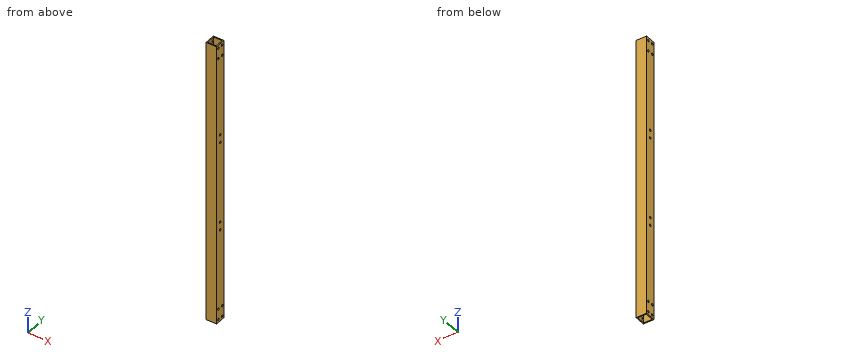
from build123d import *

# Parameters (mm, degrees)
SKETCH_1_W          = 20
SKETCH_1_H          = 20
SKETCH_1_W_2        = 16
SKETCH_1_H_2        = 16
EXTRUDE_1_DEPTH     = 560
SKETCH_2_W          = 20
SKETCH_2_H          = 20
CUT_EXTRUDE_1_DEPTH = 10
SKETCH_3_R          = 2.1
SKETCH_3_R_2        = 2.035272785
CUT_EXTRUDE_2_DEPTH = 551.454357781
SKETCH_4_R          = 2.1
CUT_EXTRUDE_3_DEPTH = 551.454357781


with BuildPart() as part:
    # 草图1 → 凸台-拉伸1 (new body)
    with BuildSketch(Plane.XY):
        Rectangle(SKETCH_1_W, SKETCH_1_H)
        Rectangle(SKETCH_1_W_2, SKETCH_1_H_2, mode=Mode.SUBTRACT)
    extrude(amount=EXTRUDE_1_DEPTH)

    # 草图2 → 切除-拉伸1 (cut)
    with BuildSketch(Plane(origin=(0, 0, 0), x_dir=(-1, 0, 0), z_dir=(0, 0, -1))):
        Rectangle(SKETCH_2_W, SKETCH_2_H)
    cut_extrude_1 = extrude(amount=-CUT_EXTRUDE_1_DEPTH, mode=Mode.SUBTRACT)

    # 镜向1: 切除-拉伸1 across plane
    add(cut_extrude_1.mirror(Plane(origin=(-40, 280, 280), x_dir=(1, 0, 0), z_dir=(0, 0, 1))), mode=Mode.SUBTRACT)

    # 草图3 → 切除-拉伸2 (cut, through all)
    with BuildSketch(Plane(origin=(10, 0, 0), x_dir=(0, 0, -1), z_dir=(1, 0, 0))):
        with Locations((-16, 5)):
            Circle(SKETCH_3_R)
        with Locations((-16, -5)):
            Circle(SKETCH_3_R_2)
        with Locations((-36, 5)):
            Circle(SKETCH_3_R)
        with Locations((-36, -5)):
            Circle(SKETCH_3_R)
        with Locations((-544, 5)):
            Circle(SKETCH_3_R)
        with Locations((-544, -5)):
            Circle(SKETCH_3_R_2)
        with Locations((-524, -5)):
            Circle(SKETCH_3_R)
        with Locations((-524, 5)):
            Circle(SKETCH_3_R)
    extrude(amount=-CUT_EXTRUDE_2_DEPTH, mode=Mode.SUBTRACT)

    # 草图4 → 切除-拉伸3 (cut, through all)
    with BuildSketch(Plane(origin=(10, 0, 0), x_dir=(0, 0, -1), z_dir=(1, 0, 0))):
        with Locations((-187.5, 0)):
            Circle(SKETCH_4_R)
        with Locations((-202.5, 0)):
            Circle(SKETCH_4_R)
        with Locations((-357.5, 0)):
            Circle(SKETCH_4_R)
        with Locations((-372.5, 0)):
            Circle(SKETCH_4_R)
    extrude(amount=-CUT_EXTRUDE_3_DEPTH, mode=Mode.SUBTRACT)


solid = part.part
Check sheet for the modelled part. Datum: model origin and axes. Units: mm. Give positions to 0.01 mm unless a question says otherwise; leave off trailing zeros. Write each loop counter-clockwise with the first axis right and the second up, starting at its lowest first coordinate (ties: lowest second). Pieces come first, ordered by that corner, then holes. Notation, with made-up numbers: (4, 56) -> (30, 56) arc R14 ccw to (30, 83) -> close; hole circle Ø7 at (44, 19.5). An arc over 180 degrees is marked (long way). Write item = value, one per line.
Item 1: Scan lines: probe 1 along Y at (x, z) = (-9, 36); probe 2 along X at (y, z) = (3.5, 188); probe 3 along Y at (x, z) = (9.2, 202.5). Record each from-to range of solid material in increasing order. Write a range as from..to.
Output:
probe_1 = -10..-7.1, -2.9..2.9, 7.1..10
probe_2 = -10..-8, 8..10
probe_3 = -10..-2.1, 2.1..10
Item 2: Gauge pin test, flat end, axial feed: pin 1 (2.5 mm diameter, centred on y = 0, z = 357.5, fed in from +X). Record the tip position at first contact, or that the pin passes through.
Output:
pin_1 = through
Item 3: Sectioned sample at A-A on z = 338. Record the boundary of the cut face in (x, y).
Output:
outline = (-10, -10) -> (10, -10) -> (10, 10) -> (-10, 10) -> close; hole (-8, -8) -> (8, -8) -> (8, 8) -> (-8, 8) -> close
